```python
from build123d import *

# Parameters (mm, degrees)
BOSS_EXTRUDE1_DEPTH = 25.4
SKETCH3_R           = 6.35
CUT_EXTRUDE1_DEPTH  = 65.288850122
SKETCH4_R           = 2.4892
CUT_EXTRUDE2_DEPTH  = 66.068137364


with BuildPart() as part:
    # Sketch2 → Boss-Extrude1 (new body)
    with BuildSketch(Plane(origin=(0, 0, 0), x_dir=(1, 0, 0), z_dir=(0, 1, 0))):
        Polygon((0, 0), (0, 50.8), (3.175, 50.8), (3.175, 3.175), (34.925, 3.175), (34.925, 0), align=None)
    extrude(amount=BOSS_EXTRUDE1_DEPTH)

    # Sketch3 → Cut-Extrude1 (cut, through all)
    with BuildSketch(Plane(origin=(0, 0, -3.175), x_dir=(-1, 0, 0), z_dir=(0, 0, -1))):
        with Locations((-22.225, 9.525)):
            Circle(SKETCH3_R)
    extrude(amount=-CUT_EXTRUDE1_DEPTH, mode=Mode.SUBTRACT)

    # Sketch4 → Cut-Extrude2 (cut, through all)
    with BuildSketch(Plane(origin=(3.175, 0, 0), x_dir=(0, 0, -1), z_dir=(1, 0, 0))):
        with Locations((25.4, 12.7)):
            Circle(SKETCH4_R)
        with Locations((12.7, 12.7)):
            Circle(SKETCH4_R)
        with Locations((38.1, 12.7)):
            Circle(SKETCH4_R)
    extrude(amount=-CUT_EXTRUDE2_DEPTH, mode=Mode.SUBTRACT)


solid = part.part
```
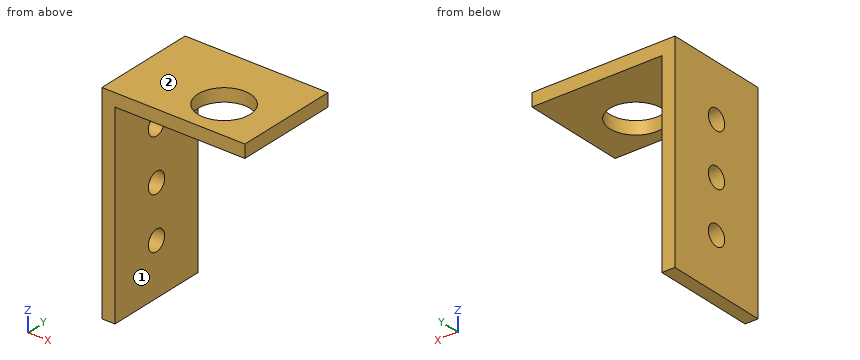
The listing builds one solid part. Answer for the finished solid, in the listing's coordinates (mm). Face numbers are marked on the shaded views. A direction names the side the tool comes from. Coordinates: 2 decimals unless noted, no trailing zeros. Order: outer loops, then holes, each group sorted by start corner. A loop starts at its lowest first (then second) coordinate and runs counter-clockwise, first axis right, second up. Notation, with made-up numbers: M 74,36 L 120,36 A11 ccw 120,47 Z; hole C -0.5,15 d3. An arc over 180 degrees is marked long. Answer as a JSON object with one key per item and string values. Group by question number.
1. Section B-B on y = 12.7 is taken. Write down the section's boundary in (x, z) (3 decimals).
2. Section A-A on z = -25.4 is taken. Write down the section's boundary in (x, y) (3 decimals), then the cut area to 3 significant figures.
3. A tool of negligible diameter and unlimited length cuts with its end or side. For the marked faces 1 and 2, from which of +Z, -Z, +X, -X, +Y, -Y can it reach the whole face along a straight path? Write none if from no direction.
4. Straight lines are drawn through the part: line 1 (Y direction, x = 2, z = -38); line 2 (X direction, y = 17.5, z = -30.5) (3 decimals); line 3 (Z direction, x = 33.5, y = 22.25) (3 decimals). For each, find the intervals that lie inside material, in ascending order.
5. Section D-D on x = 24.5 is taken. Write down the section's boundary in (y, z) (3 decimals).
6. Flat-ended cylindrical pins translate along their axes: P1, Ø6, axis at x = 30, y = 7.5, coming from the +Z side; P2, Ø4, axis at x = 10, y = 4, coming from the -Z side (3 decimals); P3, Ø6.5, axis at y = 12.7, z = -25.4, coming from the +X side (3 decimals). Find the tip coordinate at first contact, or state that the pin passes through.
7. Section C-C on x = 2 is taken. Write down the section's boundary in (y, z).
Values follow:
{
 "1": {"outline": "M 0,-50.8 L 3.175,-50.8 L 3.175,-40.589 L 0,-40.589 Z; M 0,-35.611 L 3.175,-35.611 L 3.175,-27.889 L 0,-27.889 Z; M 0,-22.911 L 3.175,-22.911 L 3.175,-15.189 L 0,-15.189 Z; M 0,-10.211 L 3.175,-10.211 L 3.175,-3.175 L 16.726,-3.175 L 16.726,0 L 0,0 Z; M 27.724,-3.175 L 34.925,-3.175 L 34.925,0 L 27.724,0 Z"},
 "2": {"outline": "M 0,0 L 3.175,0 L 3.175,10.211 L 0,10.211 Z; M 0,15.189 L 3.175,15.189 L 3.175,25.4 L 0,25.4 Z", "area": "64.8 mm2"},
 "3": {"face 1": "-Z, +X, +Y, -Y", "face 2": "+Z, +X, -X, +Y, -Y"},
 "4": {"line 1": "0 to 10.21, 15.19 to 25.4", "line 2": "0 to 3.175", "line 3": "-3.175 to 0"},
 "5": {"outline": "M 0,-3.175 L 3.597,-3.175 L 3.597,0 L 0,0 Z; M 15.453,-3.175 L 25.4,-3.175 L 25.4,0 L 15.453,0 Z"},
 "6": {"P1": "z = 0", "P2": "z = -3.175", "P3": "x = 3.175"},
 "7": {"outline": "M 0,-50.8 L 25.4,-50.8 L 25.4,0 L 0,0 Z; hole C 12.7,-38.1 d4.98; hole C 12.7,-25.4 d4.98; hole C 12.7,-12.7 d4.98"}
}
